Part model, mm, in its own coordinate system. Face numbers are marked on the shaded views. Round coordinates to 2 decimals unless told otherwise and drop trailing zeros. Order: outer loops, then holes, each group sorted by start corner. A loop starts at its lowest first (then second) coordinate and runs counter-clockwise, first axis right, second up. Notation, with made-up numbers: M 32.25,11 L 87.25,11 A19 ccw 87.25,44 Z; hole C 2,51.25 d10. An arc over 180 degrees is marked long. One line per question, with ' | ' between items.
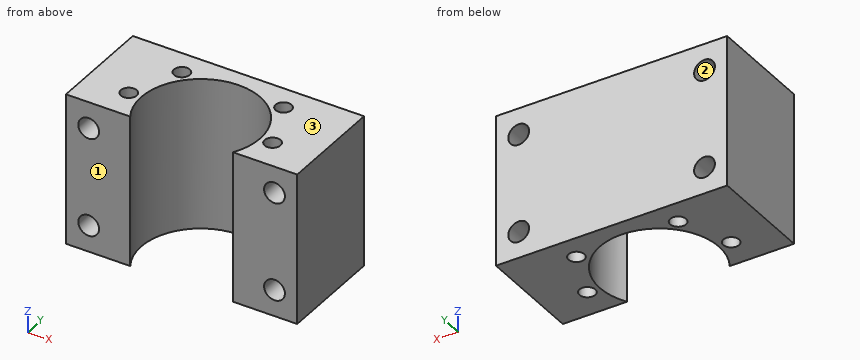
from build123d import *

# Parameters (mm, degrees)
SKETCH1_R           = 2.1
BOSS_EXTRUDE1_DEPTH = 40
SKETCH2_R           = 2.75
CUT_EXTRUDE1_DEPTH  = 50


with BuildPart() as part:
    # Sketch1 → Boss-Extrude1 (new body)
    with BuildSketch(Plane.XY):
        with BuildLine():
            Line((13.266499161, 40), (-13.266499161, 40))
            Line((-13.266499161, 40), (-27.55, 40))
            Line((-27.55, 40), (-30.55, 40))
            Line((-30.55, 40), (-30.55, 12))
            Line((-30.55, 12), (-27.55, 12))
            Line((-27.55, 12), (-13.566963551, 12))
            ThreePointArc((-13.566963551, 12), (0, 35.75), (13.566963551, 12))
            Line((13.566963551, 12), (27.55, 12))
            Line((27.55, 12), (30.55, 12))
            Line((30.55, 12), (30.55, 40))
            Line((30.55, 40), (27.55, 40))
            Line((27.55, 40), (13.266499161, 40))
        make_face()
        with Locations((-13.435028843, 33.435028843)):
            Circle(SKETCH1_R, mode=Mode.SUBTRACT)
        with Locations((19, 20)):
            Circle(SKETCH1_R, mode=Mode.SUBTRACT)
        with Locations((13.435028843, 33.435028843)):
            Circle(SKETCH1_R, mode=Mode.SUBTRACT)
        with Locations((-19, 20)):
            Circle(SKETCH1_R, mode=Mode.SUBTRACT)
    extrude(amount=-BOSS_EXTRUDE1_DEPTH)

    # Sketch2 → Cut-Extrude1 (cut)
    with BuildSketch(Plane(origin=(0, 40, 0), x_dir=(1, 0, 0), z_dir=(0, 1, 0))):
        with Locations(Location((-24.55, 33, 0), (0, 0, 270))):
            Circle(SKETCH2_R)
        with Locations(Location((-24.55, 7, 0), (0, 0, 270))):
            Circle(SKETCH2_R)
        with Locations(Location((24.55, 7, 0), (0, 0, 270))):
            Circle(SKETCH2_R)
        with Locations(Location((24.55, 33, 0), (0, 0, 270))):
            Circle(SKETCH2_R)
    extrude(amount=-CUT_EXTRUDE1_DEPTH, mode=Mode.SUBTRACT)


solid = part.part
1) Saw through at B-B (y = 24). List the corners of the cut face in (x, z).
The answers:
outline: M -30.55,-40 L -15.23,-40 L -15.23,0 L -30.55,0 Z; M 15.23,-40 L 30.55,-40 L 30.55,0 L 15.23,0 Z; hole C -24.55,-33 d5.5; hole C -24.55,-7 d5.5; hole C 24.55,-33 d5.5; hole C 24.55,-7 d5.5
2) Saw through at A-A (x = -19). List the corners of the cut face in (y, z), plus the area to 3 significant figures.
The answers:
outline: M 12,-40 L 17.9,-40 L 17.9,0 L 12,0 Z; M 22.1,-40 L 40,-40 L 40,0 L 22.1,0 Z | area: 952 mm²
3) Probe line 1 (X direction, y = 20.25, z = -17); line 2 (X direction, y = 33.75, z = -12); line 3 (Y direction, x = -19, z = -15). List the from-to ranges inside material, lowest first. Write a range as [from, to].
The answers:
line 1: x = [-30.55, -21.09], [-16.91, -15.75], [15.75, 16.91], [21.09, 30.55] | line 2: x = [-30.55, -15.51], [-11.36, -7.68], [7.68, 11.36], [15.51, 30.55] | line 3: y = [12, 17.9], [22.1, 40]
4) Two-plate mould, pull along Z, no slides. Class the marked faces 1, 2 and 3: released by +Z, released by -Z, zero draft, split by the parting line, or undercut.
The answers:
face 1: zero draft | face 2: undercut | face 3: released by +Z
5) Saw through at C-C (x = 24.55). List the corners of the cut face in (y, z), plus the area to 3 significant figures.
The answers:
outline: M 12,-40 L 40,-40 L 40,-35.75 L 12,-35.75 Z; M 12,-30.25 L 40,-30.25 L 40,-9.75 L 12,-9.75 Z; M 12,-4.25 L 40,-4.25 L 40,0 L 12,0 Z | area: 812 mm²
6) Saw through at D-D (y = 29.25). List the corners of the cut face in (x, z), plus the area to 3 significant figures.
The answers:
outline: M -30.55,-40 L -12.75,-40 L -12.75,0 L -30.55,0 Z; M 12.75,-40 L 30.55,-40 L 30.55,0 L 12.75,0 Z; hole C -24.55,-33 d5.5; hole C -24.55,-7 d5.5; hole C 24.55,-33 d5.5; hole C 24.55,-7 d5.5 | area: 1,330 mm²
